from build123d import *

# Parameters (mm, degrees)
SKETCH1_R               = 4.025
SKETCH1_R_2             = 2.125
BOSS_EXTRUDE1_DEPTH     = 2.5
SKETCH2_W               = 28.904595792
SKETCH2_H               = 55.332112
CUT_EXTRUDE1_DEPTH      = 1
CUT_EXTRUDE1_DEPTH_BACK = 6
FILLET1_R               = 4


with BuildPart() as part:
    # Sketch1 → Boss-Extrude1 (new body, symmetric)
    with BuildSketch(Plane(origin=(0, 0, 0), x_dir=(1, 0, 0), z_dir=(0, 1, 0))):
        with BuildLine():
            Line((-42.512697833, 60.569551121), (-33.895259083, 48.291939407))
            ThreePointArc((-33.895259083, 48.291939407), (-55.932258345, 18.777179671), (-56.169167779, -18.056151058))
            Line((-56.169167779, -18.056151058), (-70.449464672, -22.646697938))
            ThreePointArc((-70.449464672, -22.646697938), (-70.152324026, 23.55103891), (-42.512697833, 60.569551121))
        make_face()
        with Locations((-44.329902671, 49.233344688)):
            Circle(SKETCH1_R, mode=Mode.SUBTRACT)
        with Locations((-63, 0)):
            Circle(SKETCH1_R_2, mode=Mode.SUBTRACT)
        with Locations((-63, -15)):
            Circle(SKETCH1_R_2, mode=Mode.SUBTRACT)
        with Locations((-63, 15)):
            Circle(SKETCH1_R_2, mode=Mode.SUBTRACT)
    extrude(amount=BOSS_EXTRUDE1_DEPTH, both=True)

    # Sketch2 → Cut-Extrude1 (cut, two sides)
    with BuildSketch(Plane(origin=(0, 2.5, 0), x_dir=(1, 0, 0), z_dir=(0, 1, 0))) as cut_extrude1_sk:
        with Locations((-84.452297896, 0)):
            Rectangle(SKETCH2_W, SKETCH2_H)
    extrude(amount=CUT_EXTRUDE1_DEPTH, mode=Mode.SUBTRACT)
    extrude(cut_extrude1_sk.sketch, amount=-CUT_EXTRUDE1_DEPTH_BACK, mode=Mode.SUBTRACT)

    # Fillet1
    fillet1_edges = [part.edges().sort_by_distance(p)[0] for p in [
        (-70, 0, 22.502212941),
        (-70, 0, -24),
        (-42.512697833, 0, -60.569551121),
        (-33.895259083, 0, -48.291939407),
        (-56.169167779, 0, 18.056151058),
    ]]
    fillet(fillet1_edges, radius=FILLET1_R)


solid = part.part
Verification items for the finished model (mm, model axes). Coordinates: 2 decimals unless noted, no trailing zeros. Write each loop counter-clockwise with the first axis right and the second up, starting at its lowest first coordinate (ties: lowest second). Pieces come first, ordered by that corner, then holes. Notation, with made-up numbers: (24.25, 19.25) -> (46.25, 19.25) arc R18 ccw to (46.25, 24.25) -> close; hole circle Ø11 at (22, 58.25). An arc over 180 degrees is marked (long way). One line per item, written item: value. Start each with the question number.
Q1. Cross-section at B-B on x = -63. Enter the section's corners in (y, z) (3 decimals).
Q2. Go/stop test with a flat-tipped pin: P1, Ø10.5, axis at x = -44.33, z = -49.23, coming from the -Y side. Record where the tip stops, or that it passes through.
Q3. Cross-section at C-C on y = -0.3. Enter the section's corners in (x, z) (3 decimals), and give its area (3 significant figures).
Q4. Cross-section at A-A on z = 0. Enter the section's corners in (x, y) (3 decimals), and give its area (4 significant figures).
Q5. Cross-section at D-D on z = -15. Enter the section's corners in (x, y) (3 decimals), and give its area (3 significant figures).
Q6. Thickness scan on L1, parallel to Z at x = -64, y = 1 (3 decimals); L2, parallel to Z at x = -63, y = 1.1 (3 decimals); L3, parallel to X at y = -0.6, z = 0 (3 decimals). Record the ranges inside material, lowest first. Write a range as from..to.
Q7. Mould release check, pull along Z, two halves, no side actions. Record for faces 1 (the cylindrical face through (-65.123, -0.035, -0.093)), 2 (the flat face through (-62.28, 0.04, 20.02)), 3 (the cylindrical face through (-55.78, 0.04, -19.22)), 4 (the flat face through (-70, 0, -3)): pulls with the +Z half, pulls with the -Z half, needs draft (parallel to the pull), parting line crosses it, or undercut.
Checked values:
1. outline: (-2.5, -38.82) -> (2.5, -38.82) -> (2.5, -17.125) -> (-2.5, -17.125) -> close; (-2.5, -12.875) -> (2.5, -12.875) -> (2.5, -2.125) -> (-2.5, -2.125) -> close; (-2.5, 2.125) -> (2.5, 2.125) -> (2.5, 12.875) -> (-2.5, 12.875) -> close; (-2.5, 17.125) -> (2.5, 17.125) -> (2.5, 20.252) -> (-2.5, 20.252) -> close
2. P1: stops at y = -2.5
3. outline: (-70, -23.324) arc R4 ccw to (-69.771, -24.657) arc R74 ccw to (-45.904, -58.041) arc R4 ccw to (-40.149, -57.202) -> (-36.12, -51.462) arc R4 ccw to (-36.893, -46.042) arc R59 cw to (-57.202, 14.453) arc R4 ccw to (-59.856, 19.241) -> (-64.776, 20.823) arc R4 ccw to (-70, 17.015) -> close; hole circle Ø4.25 at (-63, -15); hole circle Ø4.25 at (-63, 0); hole circle Ø4.25 at (-63, 15); hole circle Ø8.05 at (-44.33, -49.233)
3. area: 1,030 mm²
4. outline: (-70, -2.5) -> (-65.125, -2.5) -> (-65.125, 2.5) -> (-70, 2.5) -> close; (-60.875, -2.5) -> (-59, -2.5) -> (-59, 2.5) -> (-60.875, 2.5) -> close
4. area: 33.75 mm²
5. outline: (-70, -2.5) -> (-65.125, -2.5) -> (-65.125, 2.5) -> (-70, 2.5) -> close; (-60.875, -2.5) -> (-57.061, -2.5) -> (-57.061, 2.5) -> (-60.875, 2.5) -> close
5. area: 43.4 mm²
6. L1: z = -37.148..-16.875, -13.125..-1.875, 1.875..13.125, 16.875..20.573
6. L2: z = -38.82..-17.125, -12.875..-2.125, 2.125..12.875, 17.125..20.252
6. L3: x = -70..-65.125, -60.875..-59
7. face 1: undercut
7. face 2: pulls with the +Z half
7. face 3: undercut
7. face 4: needs draft
